```python
from build123d import *

# Parameters (mm, degrees)
SKETCH_1_R          = 5
EXTRUDE_1_DEPTH     = 7.5
EXTRUDE_START       = -1.5
SKETCH_2_R          = 11
EXTRUDE_2_DEPTH     = 3.5
SKETCH_3_R          = 4
CUT_EXTRUDE_1_DEPTH = 16
SKETCH_4_R          = 1.75
CUT_EXTRUDE_2_DEPTH = 14.5
CHAMFER_1_SIZE      = 0.5


with BuildPart() as part:
    # 草图1 → 凸台-拉伸1 (new body, symmetric)
    with BuildSketch(Plane.XY):
        Circle(SKETCH_1_R)
    extrude(amount=EXTRUDE_1_DEPTH, both=True)

    # 草图2 → 凸台-拉伸2 (add)
    with BuildSketch(Plane(origin=(0, 0, -7.5), x_dir=(-1, 0, 0), z_dir=(0, 0, -1)).offset(EXTRUDE_START)):
        Circle(SKETCH_2_R)
    extrude(amount=-EXTRUDE_2_DEPTH)

    # 草图3 → 切除-拉伸1 (cut, through all)
    with BuildSketch(Plane(origin=(0, 0, -7.5), x_dir=(-1, 0, 0), z_dir=(0, 0, -1))):
        Circle(SKETCH_3_R)
    extrude(amount=-CUT_EXTRUDE_1_DEPTH, mode=Mode.SUBTRACT)

    # 草图4 → 切除-拉伸2 (cut, through all)
    with BuildSketch(Plane(origin=(0, 0, -6), x_dir=(-1, 0, 0), z_dir=(0, 0, -1))):
        with Locations((0, 8)):
            Circle(SKETCH_4_R)
        with Locations((8, 0)):
            Circle(SKETCH_4_R)
        with Locations((0, -8)):
            Circle(SKETCH_4_R)
        with Locations((-8, 0)):
            Circle(SKETCH_4_R)
    extrude(amount=-CUT_EXTRUDE_2_DEPTH, mode=Mode.SUBTRACT)

    # 倒角1
    chamfer_1_edges = [part.edges().sort_by_distance(p)[0] for p in [
        (-5, 0, -7.5),
        (-5, 0, 7.5),
        (11, 0, -2.5),
        (11, 0, -6),
    ]]
    chamfer(chamfer_1_edges, length=CHAMFER_1_SIZE)


solid = part.part
```
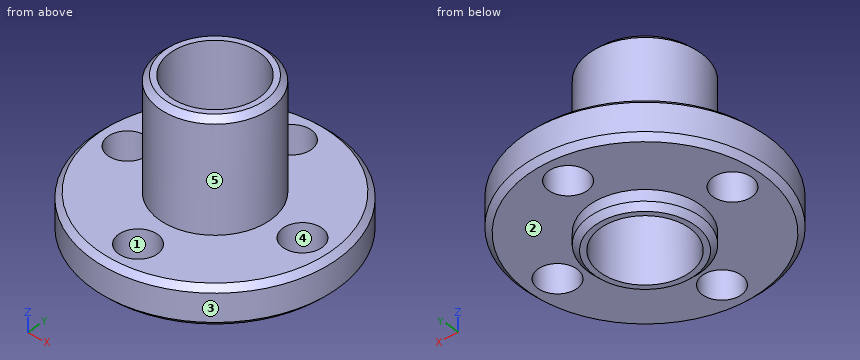
CAD build for the part. Positions are in the model's coordinates, mm. Face numbers are marked on the shaded views. A direction names the side the tool comes from. Give positions to 0.01 mm unless a question says otherwise; leave off trailing zeros. Order: outer loops, then holes, each group sorted by start corner. A loop starts at its lowest first (then second) coordinate and runs counter-clockwise, first axis right, second up. Notation, with made-up numbers: M 30,-3.5 L 41,-3.5 A9 ccw 41,10.5 Z; hole C -37.75,5 d3. An arc over 180 degrees is marked long. Put each result on its own line as item: value. Start each with the question number.
(1) Mould opens along X. For the marked faces 1, 2 and 3 say: +X half, -X half, draft (parallel to the pull), parting line (faces both ways), or undercut.
(2) Saw through at D-D, the plane z = -4. Write the cut outline in (x, y), then the cut area to 3 significant figures.
(3) Saw through at C-C, the plane z = 0.75. Write the cut outline in (x, y).
(4) Saw through at A-A, the plane y = 0. Give the number of separate pieces and of enclosed holes in the cut face, then the cut area to 3 significant figures.
(5) Drill centre lines: line 1 along Y through (x, z) = (0, -4.9); line 2 along X through (y, z) = (1.5, -3.5); line 3 along Y through (x, z) = (-0.5, -0.5). Where is each one in solid material? Low to high.
(6) Which spindle directions (+Z, -Z, +X, -X, +Y, -Y) get a long thin tool onto all of the face, cutting with end or side? Do the marked faces 4 and 5. Say none if no direction does.
(7) Flat gauge pins, fed straight in: pin 1 Ø8 at (x, z) = (-7, -2) entering from -Y; pin 2 Ø1 at (x, y) = (-5.5, -5) entering from -Z; pin 3 Ø3 at (x, y) = (0, 8) entering from +Z (3 decimals); pin 4 Ø5 at (y, z) = (-4, 2.5) entering from +X. Where does each tip first touch, or does it go through?
Check result:
1. face 1: undercut
1. face 2: draft
1. face 3: parting line
2. outline: C 0,0 d22; hole C -8,0 d3.5; hole C 0,0 d8; hole C 0,-8 d3.5; hole C 0,8 d3.5; hole C 8,0 d3.5
2. area: 291 mm2
3. outline: C 0,0 d10; hole C 0,0 d8
4. separate pieces: 4
4. enclosed holes: 0
4. area: 46.5 mm2
5. line 1: y = -11 to -9.75, -6.25 to -4, 4 to 6.25, 9.75 to 11
5. line 2: x = -10.9 to -8.9, -7.1 to -3.71, 3.71 to 7.1, 8.9 to 10.9
5. line 3: y = -4.97 to -3.97, 3.97 to 4.97
6. face 4: +Z, -Z
6. face 5: +Z
7. pin 1: stops at y = -10.55
7. pin 2: stops at z = -6
7. pin 3: passes through
7. pin 4: stops at x = 4.77
